from build123d import *

# Parameters (mm, degrees)
F0_R     = 11.15
F1_DEPTH = 7


with BuildPart() as f1:
    # F0 (on Top) → F1 (new body)
    with BuildSketch(Plane.XY):
        Polygon((12.105645, 5.433464), (0, 41.989982), (-13.375477, 5.433464), (-36.364391, -20.994991), (0, -12.173187), (36.364391, -20.994991), align=None)
        with BuildLine():
            ThreePointArc((-9.859029, 8.777217), (-10.360478, 8.179273), (-10.825715, 7.552741))
            Line((-10.825715, 7.552741), (-10.75834, 7.767064))
            Line((-10.75834, 7.767064), (-9.859029, 8.777217))
        make_face(mode=Mode.SUBTRACT)
        Circle(F0_R, mode=Mode.SUBTRACT)
    extrude(amount=F1_DEPTH)


solid = f1.part
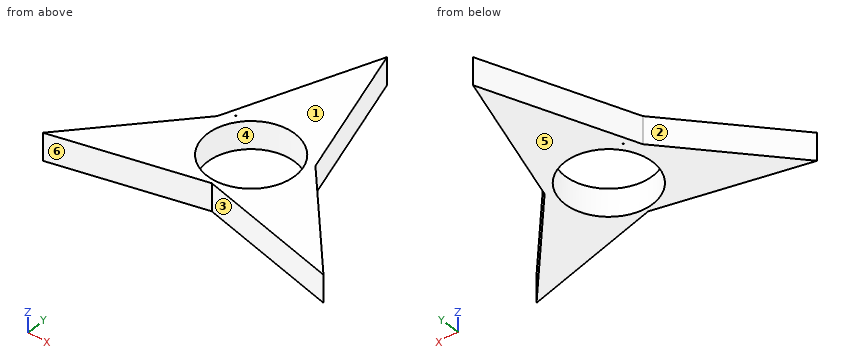
Model file for the job. Use its own axes, mm. Face numbers are marked on the shaded views. A direction names the side the tool comes from. Round coordinates to 2 decimals unless told otherwise and drop trailing zeros. Order: outer loops, then holes, each group sorted by start corner. A loop starts at its lowest first (then second) coordinate and runs counter-clockwise, first axis right, second up.
(1) Drill centre lines: line 1 (X direction, y = -2.5, z = 3); line 2 (X direction, y = 3, z = 4); line 3 (Y direction, x = 26, z = 0.5). Where is each one in solid material? Low to high.
(2) Pin check, flat tips, straight feed: pin 1 (2 mm diameter, centred on x = 26.5, z = 5, fed in from +Y); pin 2 (1 mm diameter, centred on x = -10, z = 2, fed in from -Y); pin 3 (2 mm diameter, centred on y = 18.5, z = 4.5, fed in from -X). Stop position of each tip, or through.
(3) Band-saw the part on C-C (x = -31). List the corners of the cut face in (y, z), then the cut area to 3 significant figures.
(4) Band-saw the part on A-A (y = -3). List the corners of the cut face in (x, z), then the cut area to 3 significant figures.
(5) Band-saw the part on B-B (z = 3). List the corners of the cut face in (x, y) (3 decimals), then the cut area to 3 significant figures.
(6) Pull direction X, two halves, no side cores. Call the marked faces 1, 2, 3 and 4: released by +X, released by -X, zero draft, split by the parting line, or undercut.
(7) 3-axis set-ups, long thin cutter, end or side, ignore diameter. For the marked faces 5 and 6: which of +Z, -Z, +X, -X, +Y, -Y reach the whole face in a straight line?
(8) Band-saw the part on D-D (y = -14). List the corners of the cut face in (x, z).
Verdict:
1. line 1: x = -20.28 to -10.87, 10.87 to 19.39
1. line 2: x = -15.49 to -10.74, 10.74 to 14.34
1. line 3: y = -18.48 to -9.7
2. pin 1: stops at y = -9.16
2. pin 2: stops at y = -14.72
2. pin 3: stops at x = -8.96
3. outline: (-19.69, 0) - (-14.83, 0) - (-14.83, 7) - (-19.69, 7) - close
3. area: 34.1 mm2
4. outline: (-20.71, 0) - (-10.74, 0) - (-10.74, 7) - (-20.71, 7) - close; (10.74, 0) - (19.85, 0) - (19.85, 7) - (10.74, 7) - close
4. area: 134 mm2
5. outline: (-36.364, -20.995) - (0, -12.173) - (36.364, -20.995) - (12.106, 5.433) - (0, 41.99) - (-13.375, 5.433) - close; hole circle Ø22.3 at (0, 0); hole (-10.826, 7.553) arc R13.2 cw to (-9.859, 8.777) - (-10.758, 7.767) - close
5. area: 1,050 mm2
6. face 1: zero draft
6. face 2: released by -X
6. face 3: undercut
6. face 4: undercut
7. face 5: -Z, +X, -X, +Y, -Y
7. face 6: +Z, -Z, -Y
8. outline: (-30.28, 0) - (-7.53, 0) - (-7.53, 7) - (-30.28, 7) - close; (7.53, 0) - (29.94, 0) - (29.94, 7) - (7.53, 7) - close
